Input: dimensioned drawing with shaded views. Units: mm. Origin: part minimum x, y, z. Give positions to 0.01 mm unless a question says otherwise; leave off trailing zeros. Order: outer loops, then holes, each group sorted by start corner. A loop starts at its lowest first (then second) coordinate and runs counter-clockwise, first axis right, second up.
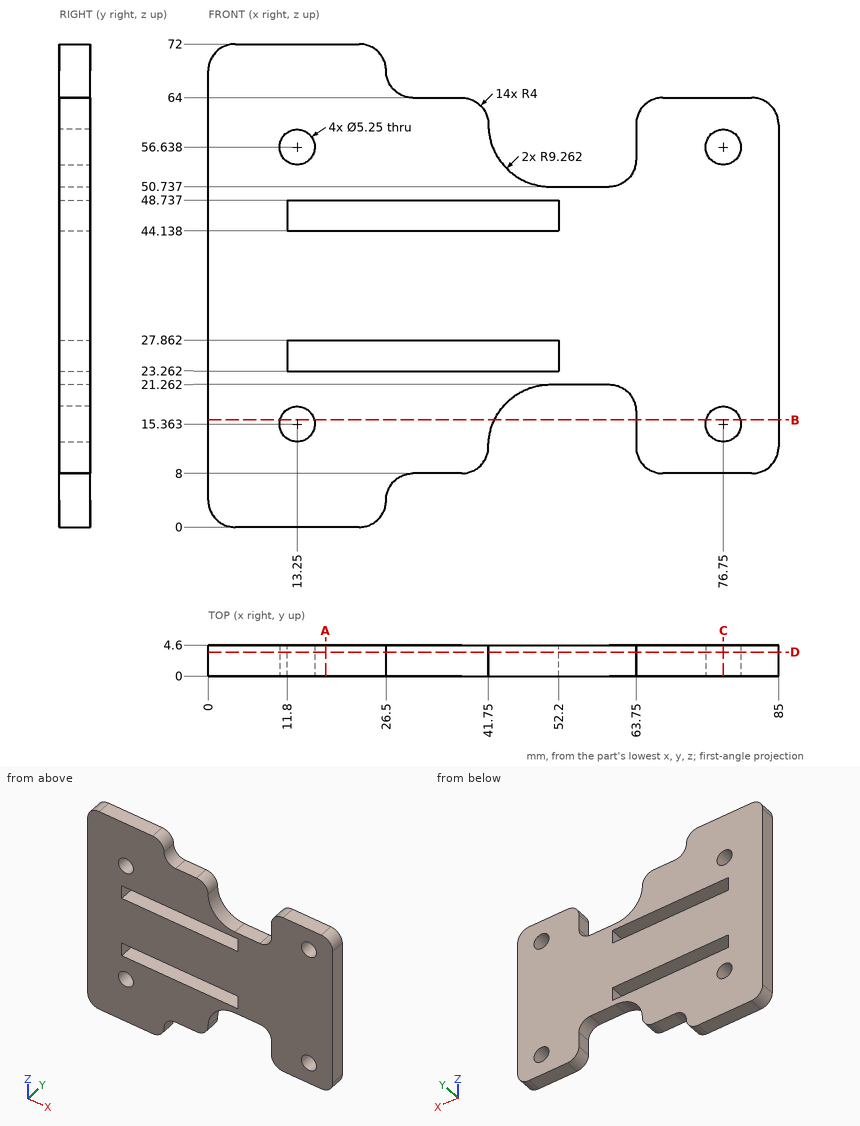
1) First-contact query: P1, Ø3, axis at x = 76.75, z = 56.64, coming from the +Y side; P2, Ø1, axis at x = 20.5, y = 4, coming from the -Z side; P3, Ø1.4, axis at x = 75.5, y = 3, coming from the -Z side; P4, Ø1.4, axis at x = 55.5, y = 3.5, coming from the +Z side. Flat tips, straight axial feed; report the tip coordinate or a pass-through.
2) Cut plane B-B (z = 16). Return the cut outline in (x, y), then the cut area to 3 significant figures.
3) Cut plane D-D (y = 3.55). Count the separate pieces of the cut face and the enclosed holes in it, then the cut area to 3 significant figures.
4) Cut plane C-C (x = 76.75). Return the cut outline in (y, z).
5) Cut plane A-A (x = 17.5). Return the cut outline in (y, z).
6) Line query: probe 1 along Z at (x, y) = (13.25, 3.2); probe 2 along Z at (x, y) = (16, 1.3); probe 3 along Z at (x, y) = (76.75, 1.7). Output: solid intervals per line, ascending.
Geometry says:
1. P1: passes through
1. P2: stops at z = 0
1. P3: stops at z = 8
1. P4: stops at z = 50.74
2. outline: (0, 0) - (10.7, 0) - (10.7, 4.6) - (0, 4.6) - close; (15.8, 0) - (42.66, 0) - (42.66, 4.6) - (15.8, 4.6) - close; (63.75, 0) - (74.2, 0) - (74.2, 4.6) - (63.75, 4.6) - close; (79.3, 0) - (85, 0) - (85, 4.6) - (79.3, 4.6) - close
2. area: 247 mm2
3. separate pieces: 1
3. enclosed holes: 6
3. area: 4,160 mm2
4. outline: (0, 8) - (4.6, 8) - (4.6, 12.74) - (0, 12.74) - close; (0, 17.99) - (4.6, 17.99) - (4.6, 54.01) - (0, 54.01) - close; (0, 59.26) - (4.6, 59.26) - (4.6, 64) - (0, 64) - close
5. outline: (0, 0) - (4.6, 0) - (4.6, 23.26) - (0, 23.26) - close; (0, 27.86) - (4.6, 27.86) - (4.6, 44.14) - (0, 44.14) - close; (0, 48.74) - (4.6, 48.74) - (4.6, 72) - (0, 72) - close
6. probe 1: z = 0 to 12.74, 17.99 to 23.26, 27.86 to 44.14, 48.74 to 54.01, 59.26 to 72
6. probe 2: z = 0 to 23.26, 27.86 to 44.14, 48.74 to 72
6. probe 3: z = 8 to 12.74, 17.99 to 54.01, 59.26 to 64
